Input: part model. Units: mm. Frame: model coordinates. Give positions to 0.01 mm unless a question says otherwise; leave off trailing zeros. Write each loop counter-clockwise with the first axis right and the second up, starting at its lowest first coordinate (ties: lowest second). Pieces come first, ordered by that corner, then holes.
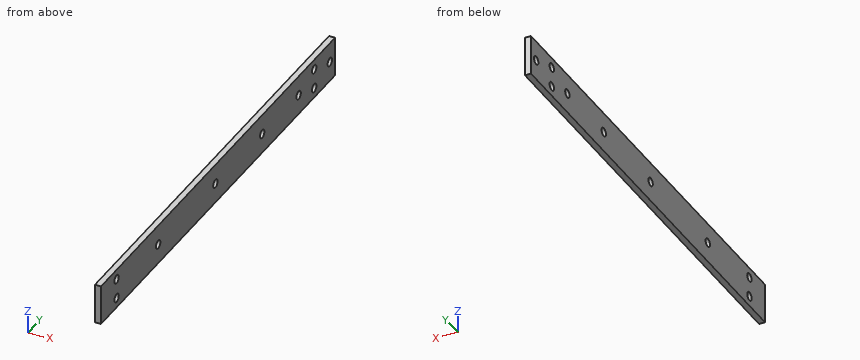
```python
from build123d import *

# Parameters (mm, degrees)
SKETCH_1_W      = 225
SKETCH_1_H      = 20
SKETCH_1_R      = 2.1
EXTRUDE_1_DEPTH = 3


with BuildPart() as part:
    # 草图1 → 凸台-拉伸1 (new body)
    with BuildSketch(Plane(origin=(-39, 0, 0), x_dir=(0, -1, 0), z_dir=(-1, 0, 0))):
        with Locations((-107.5, 10)):
            Rectangle(SKETCH_1_W, SKETCH_1_H)
        with Locations(Location((-215, 10, 0), (0, 0, 270))):
            Circle(SKETCH_1_R, mode=Mode.SUBTRACT)
        with Locations(Location((-200, 15, 0), (0, 0, 270))):
            Circle(SKETCH_1_R, mode=Mode.SUBTRACT)
        with Locations(Location((-185, 10, 0), (0, 0, 270))):
            Circle(SKETCH_1_R, mode=Mode.SUBTRACT)
        with Locations(Location((-10, 5, 0), (0, 0, 270))):
            Circle(SKETCH_1_R, mode=Mode.SUBTRACT)
        with Locations(Location((-10, 15, 0), (0, 0, 270))):
            Circle(SKETCH_1_R, mode=Mode.SUBTRACT)
        with Locations(Location((-200, 5, 0), (0, 0, 270))):
            Circle(SKETCH_1_R, mode=Mode.SUBTRACT)
        with Locations(Location((-150, 10, 0), (0, 0, 270))):
            Circle(SKETCH_1_R, mode=Mode.SUBTRACT)
        with Locations(Location((-105, 10, 0), (0, 0, 270))):
            Circle(SKETCH_1_R, mode=Mode.SUBTRACT)
        with Locations(Location((-50, 10, 0), (0, 0, 270))):
            Circle(SKETCH_1_R, mode=Mode.SUBTRACT)
    extrude(amount=-EXTRUDE_1_DEPTH)


solid = part.part
```
Q1. Section B-B, the plane z = 10. Return the cut outline in (x, y), then the cut area to 3 significant figures.
Q2. Material intervals for line 1 along Y through (x, z) = (-38.1, 5); line 2 along Y through (x, z) = (-37.9, 10); line 3 along Z through (x, y) = (-36.9, 200), sorted ascending.
Q3. Pin query (flat end, axial travel): pin 1 (2.5 mm diameter, centred on y = 200, z = 15, fed in from -X). Return the tip coordinate at first contact, or that it passes through.
Q4. Section D-D, the plane x = -38.35. Give the number of separate pieces and of enclosed holes in the cut face, then the cut area to 3 significant figures.
Q5. Section C-C, the plane y = 10. Return the cut outline in (x, z).
Q6. Section A-A, the plane y = 215. Return the cut outline in (x, z), then the cut area to 3 significant figures.
Solutions:
1. outline: (-39, -5) - (-36, -5) - (-36, 47.9) - (-39, 47.9) - close; (-39, 52.1) - (-36, 52.1) - (-36, 102.9) - (-39, 102.9) - close; (-39, 107.1) - (-36, 107.1) - (-36, 147.9) - (-39, 147.9) - close; (-39, 152.1) - (-36, 152.1) - (-36, 182.9) - (-39, 182.9) - close; (-39, 187.1) - (-36, 187.1) - (-36, 212.9) - (-39, 212.9) - close; (-39, 217.1) - (-36, 217.1) - (-36, 220) - (-39, 220) - close
1. area: 612 mm2
2. line 1: y = -5 to 7.9, 12.1 to 197.9, 202.1 to 220
2. line 2: y = -5 to 47.9, 52.1 to 102.9, 107.1 to 147.9, 152.1 to 182.9, 187.1 to 212.9, 217.1 to 220
2. line 3: z = 0 to 2.9, 7.1 to 12.9, 17.1 to 20
3. pin 1: passes through
4. separate pieces: 1
4. enclosed holes: 9
4. area: 4,380 mm2
5. outline: (-39, 0) - (-36, 0) - (-36, 2.9) - (-39, 2.9) - close; (-39, 7.1) - (-36, 7.1) - (-36, 12.9) - (-39, 12.9) - close; (-39, 17.1) - (-36, 17.1) - (-36, 20) - (-39, 20) - close
6. outline: (-39, 0) - (-36, 0) - (-36, 7.9) - (-39, 7.9) - close; (-39, 12.1) - (-36, 12.1) - (-36, 20) - (-39, 20) - close
6. area: 47.4 mm2
